Autodesk Inventor part; units mm, degrees
ref_plane "YZ Plane" through (0, 0, 0) normal (1, 0, 0) x (0, 1, 0)
ref_plane "XZ Plane" through (0, 0, 0) normal (0, 1, 0) x (-1, 0, 0)
ref_plane "XY Plane" through (0, 0, 0) normal (0, 0, 1) x (1, 0, 0)
sketch "Sketch1" plane through (0, 0, 0) normal (0, 0, 1) x (1, 0, 0)
  line L0 (0, 20.7105) -> (0, 20.7105)
  line L1 (4, 16.7105) -> (4, 14.6095)
  line L2 (0, -20.7105) -> (0, -20.7105)
  line L3 (-4, -16.7105) -> (-4, 1.4635)
  line L4 (-4, 20.7105) -> (0, 20.7105) construction
  line L5 (0, 20.7105) -> (0, 0) construction
  line L6 (0, 0) -> (-4, 0) construction
  line L7 (-4, 0) -> (-4, 20.7105) construction
  arc A0 (4, 16.7105) -> (0, 20.7105) centre (0, 16.7105) ccw
  arc A1 (0, 20.7105) -> (-4, 16.7105) centre (0, 16.7105) ccw
  arc A2 (-4, -16.7105) -> (0, -20.7105) centre (0, -16.7105) ccw
  arc A3 (0, -20.7105) -> (4, -16.7105) centre (0, -16.7105) ccw
  line L8 (-4, 1.4635) -> (4, 14.6095)
  line L9 (-4, 1.4635) -> (-4, 16.7105)
  line L10 (4, 14.6095) -> (4, -16.7105)
  dimension "d0" = 4
  dimension "d6" = 33.421
extrude "Extrusion2" add sketch "Sketch1" along normal mid plane 5 contours L1 L8 L9 A1 A0
extrude "Extrusion3" add sketch "Sketch1" along normal mid plane 10 contours L10 A3 A2 L3 L8
fillet "Fillet1" radius 2 4 edges at (4, 14.6095, -3.75) (-4, 1.4635, -3.75) (4, 14.6095, 3.75) (-4, 1.4635, 3.75)
sketch "Sketch3" plane through (0, 0, -5) normal (0, 0, -1) x (-1, 0, 0)
  arc A0 (-4, -16.7105) -> (4, -16.7105) centre (0, -16.7105) ccw
  arc A1 (4, 16.7105) -> (-4, 16.7105) centre (0, 16.7105) ccw
  line L0 (-4, 7.4758) -> (-4, 16.7105)
  arc A2 (-0.2915, 8.5155) -> (-4, 7.4758) centre (-2, 7.4758) ccw
  line L1 (3.7085, 1.9425) -> (-0.2915, 8.5155)
  arc A3 (4, 0.9028) -> (3.7085, 1.9425) centre (2, 0.9028) ccw
  line L2 (4, 0.9028) -> (4, 16.7105)
  point P0 (0, 0)
hole "Hole2" at (0, 16.7105, -5) at (0, -16.7105, -5) direction (0, 0, 1) diameter 3.4 end through all
sketch "Sketch4" plane through (0, 0, -2.5) normal (0, 0, -1) x (-1, 0, 0)
  circle A0 centre (0, 16.7105) radius 1.7
  arc A1 (4, 16.7105) -> (-4, 16.7105) centre (0, 16.7105) ccw
  line L0 (-4, 7.4758) -> (-4, 16.7105)
  arc A2 (-0.2915, 8.5155) -> (-4, 7.4758) centre (-2, 7.4758) ccw
  line L1 (3.7085, 1.9425) -> (-0.2915, 8.5155)
  arc A3 (4, 0.9028) -> (3.7085, 1.9425) centre (2, 0.9028) ccw
  line L2 (4, 0.9028) -> (4, 16.7105)
  point P0 (0, 0)
extrude "Extrusion4" cut sketch "Sketch4" against normal up to surface (2.5 mm away)
equation "\"d6\" = LengthJ"
properties part number "F"
Design review of the part built by this model. Coordinates are the model's own, in mm. A direction names the side the tool comes from. Give positions to 0.01 mm unless a question says otherwise; leave off trailing zeros. Write each loop counter-clockwise with the first axis right and the second up, starting at its lowest first coordinate (ties: lowest second). Pieces come first, ordered by that corner, then holes. Notation, with made-up numbers: M 20.25,10.25 L 77.25,10.25 A15 cw 77.25,31.25 Z; hole C 32.5,44.25 d5. An arc over 180 degrees is marked long. Return JSON: item names as keys, results as strings. Group by question number.
Item 1: Clearance check with flat-ended pins moving along their axes: pin 1 Ø2 at (x, z) = (-0.5, 4) entering from +Y; pin 2 Ø1 at (x, z) = (-2, -3) entering from -Y; pin 3 Ø1.5 at (x, z) = (0.5, -2) entering from +Y. State where each tip first meets the part, or that it passes through.
Item 2: Take a section at B-B (z = 0.75). Give the boundary of the cut face in (x, y), plus the area to 3 significant figures.
Item 3: Wall thickness on line 1 along Y through (x, z) = (0, 1.9); line 2 along Z through (x, y) = (0.5, 13); line 3 along X through (y, z) = (17.5, 1): over which ranges is each line inside the solid? List them lowest first.
Item 4: Take a section at A-A (z = -1.25). Give the boundary of the cut face in (x, y), plus the area to 3 significant figures.
Item 5: The part is to be moulded in two halves that separate along Y. For faces 1 (the cylindrical face through (-0.51, -15.09, 0.07)), 2 (the cylindrical face through (-0.07, 15.01, 1.27)), 3 (the flat face through (-4, -4, 0)), 4 (the cylindrical face through (-3.924, 1.45, 3.768)), say which applies: pulls with the +Y half, pulls with the -Y half, needs draft (parallel to the pull), parting line crosses it, or undercut.
Item 6: Tool access review of faces 5 (the cylindrical face through (-3.928, 1.435, -1.268)), 6 (the flat face through (-1.74, 5.18, 3.73)), 7 (the flat face through (0, -5, -5)), 8 (the cylindrical face through (2.575, 9.391, 3.768)), 9 (the cylindrical face through (-0.09, -20.71, 0.07)): name each direction out of +Z, -Z, +X, -X, +Y, -Y from which nothing blocks a thin tool from reaching the whole face with its end or side.
Item 7: Take a section at D-D (y = 9). Give the boundary of the cut face in (x, z), plus the area to 3 significant figures.
Item 8: Take a section at C-C (x = -0.5). Give the boundary of the cut face in (y, z).
Return value:
{
 "1": {"pin 1": "stops at y = 8.8", "pin 2": "stops at y = -20.42", "pin 3": "stops at y = 9.33"},
 "2": {"outline": "M -4,-16.71 A4 ccw 4,-16.71 L 4,16.71 A4 ccw -4,16.71 Z; hole C 0,-16.71 d3.4; hole C 0,16.71 d3.4", "area": "299 mm2"},
 "3": {"line 1": "y = -20.71 to -18.41, -15.01 to 15.01, 18.41 to 20.71", "line 2": "z = 0 to 2.5", "line 3": "x = -3.92 to -1.51, 1.51 to 3.92"},
 "4": {"outline": "M -4,-16.71 A4 ccw 4,-16.71 L 4,7.48 A2 ccw 0.29,8.52 L -3.71,1.94 A2 ccw -4,0.9 Z; hole C 0,-16.71 d3.4", "area": "205 mm2"},
 "5": {"face 1": "undercut", "face 2": "undercut", "face 3": "needs draft", "face 4": "pulls with the +Y half"},
 "6": {"face 5": "-Z, -X, +Y", "face 6": "+Z, -X, +Y", "face 7": "-Z, +X, -X, +Y, -Y", "face 8": "+Z, +Y", "face 9": "+Z, -Z, -Y"},
 "7": {"outline": "M -4,0 L 0.71,0 L 0.71,-5 L 3.29,-5 L 3.29,0 L 4,0 L 4,2.5 L 3.29,2.5 L 3.29,5 L 0.71,5 L 0.71,2.5 L -4,2.5 Z", "area": "39.4 mm2"},
 "8": {"outline": "M -20.68,-5 L -18.34,-5 L -18.34,5 L -20.68,5 Z; M -15.09,-5 L 7.21,-5 L 7.21,0 L 15.09,0 L 15.09,2.5 L 7.21,2.5 L 7.21,5 L -15.09,5 Z; M 18.34,0 L 20.68,0 L 20.68,2.5 L 18.34,2.5 Z"}
}
